```python
from build123d import *

# Parameters (mm, degrees)
F0_W          = 109
F0_H          = 179
F1_DEPTH      = 3
F2_R          = 10
F3_W          = 109
F3_H          = 76
F4_DEPTH      = 25
F4_DEPTH_BACK = 7


with BuildPart() as f1:
    # F0 (on Front) → F1 (new body)
    with BuildSketch(Plane.XZ):
        Rectangle(F0_W, F0_H)
    extrude(amount=F1_DEPTH)

    # F2
    f2_edges = [f1.edges().sort_by_distance(p)[0] for p in [
        (54.5, -1.5, 89.5),
        (-54.5, -1.5, 89.5),
        (54.5, -1.5, -89.5),
        (-54.5, -1.5, -89.5),
    ]]
    fillet(f2_edges, radius=F2_R)

    # F3 (on face) → F4 (join, two sides)
    with BuildSketch(Plane.XZ.offset(3)) as f4_sk:
        with Locations((0, -27.5)):
            Rectangle(F3_W, F3_H)
    extrude(amount=F4_DEPTH)
    extrude(f4_sk.sketch, amount=-F4_DEPTH_BACK)


solid = f1.part
```
Geometry check sheet. Reference: the model listing, model coordinates, mm. A direction names the side the tool comes from. Coordinates: 2 decimals unless noted, no trailing zeros. Write each loop counter-clockwise with the first axis right and the second up, starting at its lowest first coordinate (ties: lowest second). Pieces come first, ordered by that corner, then holes. Notation, with made-up numbers: M 66.5,-24 L 114.5,-24 A15 ccw 114.5,-15 Z; hole C 18.25,-24 d10. An arc over 180 degrees is marked long. Answer as a JSON object with one key per item and string values.
1. Tool access check on faces 1 (the flat face through (-1, 2, 10.5)), 2 (the flat face through (-1, -3, 51)), 3 (the flat face through (-1, 2, -65.5)), 4 (the flat face through (-1, -3, -77)). Record the directions out of +Z, -Z, +X, -X, +Y, -Y that give a thin tool (end or side, any length) a straight path to the whole face; none if there is none.
Answers below:
{"face 1": "+Z, +X, -X, +Y", "face 2": "+Z, +X, -X, -Y", "face 3": "-Z, +X, -X, +Y", "face 4": "-Z, +X, -X, -Y"}
2. Section check C-C, the plane z = 33. Enter the section's corners in (x, y).
Answers below:
{"outline": "M -54.5,-3 L 54.5,-3 L 54.5,0 L -54.5,0 Z"}
3. Section check A-A, the plane x = 21. Enter the section's corners in (y, z), plus the area to 3 significant figures.
Answers below:
{"outline": "M -28,-65.5 L -3,-65.5 L -3,-89.5 L 0,-89.5 L 0,-65.5 L 4,-65.5 L 4,10.5 L 0,10.5 L 0,89.5 L -3,89.5 L -3,10.5 L -28,10.5 Z", "area": "2,740 mm²"}
4. Scan lines: L1, parallel to Z at x = 15.5, y = -6.5; L2, parallel to Y at x = 26, z = 70.5. Record each from-to range of solid material in increasing order.
Answers below:
{"L1": "z = -65.5 to 10.5", "L2": "y = -3 to 0"}
5. Section check B-B, the plane y = -11.5. Enter the section's corners in (x, z), plus the area to 3 significant figures.
Answers below:
{"outline": "M -54.5,-65.5 L 54.5,-65.5 L 54.5,10.5 L -54.5,10.5 Z", "area": "8,280 mm²"}
6. Go/stop test with flat-tipped pins: pin 1 Ø8 at (x, y) = (16, -8) entering from -Z; pin 2 Ø7 at (x, z) = (-2.5, -72.5) entering from -Y; pin 3 Ø12 at (x, z) = (-18, -82) entering from +Y. Record where each tip stops, or that it passes through.
Answers below:
{"pin 1": "stops at z = -65.5", "pin 2": "stops at y = -3", "pin 3": "stops at y = 0"}
